Design review of the part built by this model. Coordinates are the model's own, in mm. Coordinates: 2 decimals unless noted, no trailing zeros. Loops run counter-clockwise (first coordinate to the right, second up) from the corner with the lowest first, then second, coordinate; pieces in that order, holes last. Notation, with made-up numbers: M 62.25,38 L 89.25,38 A30 ccw 89.25,68 Z; hole C 47.5,67.25 d9. An arc over 180 degrees is marked long. One line per item, written item: value.
```python
from build123d import *

# Parameters (mm, degrees)
SKETCH1_R           = 0.227761077
BOSS_EXTRUDE1_DEPTH = 1
SKETCH4_R           = 0.251968504
CUT_EXTRUDE1_DEPTH  = 10


with BuildPart() as part:
    # Sketch1 → Boss-Extrude1 (new body)
    with BuildSketch(Plane.XY):
        with BuildLine():
            Line((3.44382586, -27.356132879), (3.44382586, -66.756132879))
            ThreePointArc((3.44382586, -66.756132879), (3.94382586, -67.256132879), (4.44382586, -66.756132879))
            Line((4.44382586, -66.756132879), (4.44382586, -27.356132879))
            Line((4.44382586, -27.356132879), (4.44382586, -26.541134356))
            Line((4.44382586, -26.541134356), (3.44382586, -26.541134356))
            Line((3.44382586, -26.541134356), (3.44382586, -27.356132879))
        make_face()
        with Locations((3.94382586, -66.756132879)):
            Circle(SKETCH1_R, mode=Mode.SUBTRACT)
    extrude(amount=BOSS_EXTRUDE1_DEPTH)

    # Sketch4 → Cut-Extrude1 (cut)
    with BuildSketch(Plane(origin=(4.44382586, 0, 0), x_dir=(0, 0, -1), z_dir=(1, 0, 0))):
        with Locations((-0.5, -27.356132879)):
            Circle(SKETCH4_R)
    extrude(amount=-CUT_EXTRUDE1_DEPTH, mode=Mode.SUBTRACT)


solid = part.part
```
(1) To check wall thickness, follow line 1 along Y through (x, z) = (4.1, 0.7); line 2 along Y through (x, z) = (3.8, 0.35) (3 decimals); line 3 along Y through (x, z) = (4, 0.1). State the ranges of each line that lie inside material, in increasing order. Write a range as [from, to].
Reply:
line 1: y = [-67.23, -66.92], [-66.59, -27.51], [-27.2, -26.54]
line 2: y = [-67.235, -66.933], [-66.58, -27.559], [-27.154, -26.541]
line 3: y = [-67.25, -66.98], [-66.54, -26.54]
(2) Mouldability with a two-part tool opening along Y and no side actions: class faces 1 (the flat face through (4, -26.541, 0.5)), 2 (the cylindrical face through (3.933, -67.256, 0.493)), 3 (the flat face through (4, -47, 1)) as released by +Y, released by -Y, zero draft, split by the parting line, or undercut.
Reply:
face 1: released by +Y
face 2: released by -Y
face 3: zero draft
(3) We need section B-B on x = 4. State the section outline as (y, z) points, then the cut area to 3 significant figures.
Reply:
outline: M -67.25,0 L -66.98,0 L -66.98,1 L -67.25,1 Z; M -66.54,0 L -26.54,0 L -26.54,1 L -66.54,1 Z; hole C -27.36,0.5 d0.5
area: 40.1 mm2
(4) We need section A-A on z = 0.5. State the section outline as (x, y) points, then the cut area to 3 significant figures.
Reply:
outline: M 3.44,-66.76 A0.5 ccw 4.44,-66.76 L 4.44,-27.61 L 3.44,-27.61 Z; M 3.44,-27.1 L 4.44,-27.1 L 4.44,-26.54 L 3.44,-26.54 Z; hole C 3.94,-66.76 d0.46
area: 39.9 mm2
